from build123d import *

# Parameters (mm, degrees)
F1_DEPTH = 0.3175
F3_DEPTH = 304.8
F5_DEPTH = 304.8


with BuildPart() as f1:
    # F0 (on Front) → F1 (new body)
    with BuildSketch(Plane.XZ):
        Polygon((105.5624, -50.8), (152.4, -50.8), (152.4, -12.7), (-152.4, -12.7), (-152.4, -50.8), (-105.56875, -50.8), (-105.56875, -25.4), (-97.6376, -25.4), (-97.6376, -50.8), (-54.7624, -50.8), (-54.7624, -25.4), (-46.83125, -25.4), (-46.83125, -50.8), (-3.9624, -50.8), (-3.9624, -25.4), (3.9624, -25.4), (3.9624, -50.8), (46.8376, -50.8), (46.8376, -25.4), (54.7624, -25.4), (54.7624, -50.8), (97.6376, -50.8), (97.6376, -25.4), (105.5624, -25.4), align=None)
    extrude(amount=F1_DEPTH)

    # F2 (on face) → F3 (join)
    with BuildSketch(Plane(origin=(-152.4, 0, 0), x_dir=(0, -1, 0), z_dir=(-1, 0, 0))):
        Polygon((0, -12.7), (0.3175, -12.7), (54.199037, 41.181537), (54.040287, 41.340287), align=None)
    extrude(amount=-F3_DEPTH)

    # F4 (on face) → F5 (join)
    with BuildSketch(Plane(origin=(-152.4, 0, 0), x_dir=(0, -1, 0), z_dir=(-1, 0, 0))):
        Polygon((72.159549, 23.221024), (54.199037, 41.181537), (53.97453, 40.95703), (71.935043, 22.996518), align=None)
    extrude(amount=-F5_DEPTH)


solid = f1.part
The listing builds one solid part. Answer for the finished solid, in the listing's coordinates (mm). A direction names the side the tool comes from. Coordinates: 2 decimals unless noted, no trailing zeros. Write each loop counter-clockwise with the first axis right and the second up, starting at its lowest first coordinate (ties: lowest second). Pieces come first, ordered by that corner, then holes. Notation, with made-up numbers: (-23, 46) - (23, 46) arc R22 ccw to (23, 52) - close; hole circle Ø7 at (50.25, 44.25). An arc over 180 degrees is marked (long way). Put each result on its own line as item: value.
1. Flat-ended cylindrical pins translate along their axes: pin 1 Ø6 at (x, y) = (-1, -57) entering from -Z; pin 2 Ø5 at (x, y) = (-68, -12) entering from -Z; pin 3 Ø5 at (x, z) = (118, 2) entering from -Y. Find the tip coordinate at first contact, or state that the pin passes through.
Answer sheet:
pin 1: stops at z = 34.93
pin 2: stops at z = -3.52
pin 3: stops at y = -17.52
2. A tool of negligible diameter and unlimited length cuts with its end or side. For faces 1 (the face through (-2, 0, -23)), 2 (the face through (-2.13, -62.83, 32.1)), from which of +Z, -Z, +X, -X, +Y, -Y can it reach the whole face along a straight path? Write none if from no direction.
Answer sheet:
face 1: +Z, -Z, +X, -X, +Y
face 2: -Z, +X, -X
3. The part is cut by section C-C on z = 29. Give the vertices of the cut face in (x, y).
Answer sheet:
outline: (-152.4, -66.38) - (152.4, -66.38) - (152.4, -65.93) - (-152.4, -65.93) - close; (-152.4, -42.02) - (152.4, -42.02) - (152.4, -41.7) - (-152.4, -41.7) - close
4. Determine the mould class of faces 3 (the face through (-2.1, -27.4, 14.7)), 4 (the face through (-2, -0.318, -23)), 5 (the face through (-2.13, -26.77, 13.75)) for opening direction Y: pulls with the +Y half, pulls with the -Y half, needs draft (parallel to the pull), parting line crosses it, or undercut.
Answer sheet:
face 3: pulls with the +Y half
face 4: pulls with the -Y half
face 5: undercut
5. Find the intervals of material crossed by line 1 along Y through (x, z) = (-81.5, -43); line 2 along Z through (x, y) = (-32.5, -54); line 3 along Y through (x, z) = (-118, 32.5), in increasing order. Write a range as from..to.
Answer sheet:
line 1: y = -0.32..0
line 2: z = 40.93..41.3
line 3: y = -62.88..-62.43, -45.52..-45.2
6. The part is cut by section B-B on x = 101.5. Give the vertices of the cut face in (y, z), plus the area to 3 significant figures.
Answer sheet:
outline: (-72.16, 23.22) - (-71.94, 23) - (-53.97, 40.96) - (-0.32, -12.7) - (-0.32, -25.4) - (0, -25.4) - (0, -12.7) - (-54.04, 41.34) - close
area: 29.2 mm^2
7. The part is cut by section D-D on x = -17.5. Give the vertices of the cut face in (y, z).
Answer sheet:
outline: (-72.16, 23.22) - (-71.94, 23) - (-53.97, 40.96) - (-0.32, -12.7) - (-0.32, -50.8) - (0, -50.8) - (0, -12.7) - (-54.04, 41.34) - close
8. The part is cut by section A-A on z = -30. Give the vertices of the cut face in (x, y), plus the area to 3 significant figures.
Answer sheet:
outline: (-152.4, -0.32) - (-105.57, -0.32) - (-105.57, 0) - (-152.4, 0) - close; (-97.64, -0.32) - (-54.76, -0.32) - (-54.76, 0) - (-97.64, 0) - close; (-46.83, -0.32) - (-3.96, -0.32) - (-3.96, 0) - (-46.83, 0) - close; (3.96, -0.32) - (46.84, -0.32) - (46.84, 0) - (3.96, 0) - close; (54.76, -0.32) - (97.64, -0.32) - (97.64, 0) - (54.76, 0) - close; (105.56, -0.32) - (152.4, -0.32) - (152.4, 0) - (105.56, 0) - close
area: 84.2 mm^2
